Source: CAD feature listing. Evaluate the final solid. Frame: model axes, mm. Give positions to 0.01 mm unless a question says otherwise; leave off trailing zeros. Order: outer loops, then holes, each group sorted by start corner. A loop starts at its lowest first (then second) coordinate and runs counter-clockwise, first axis right, second up.
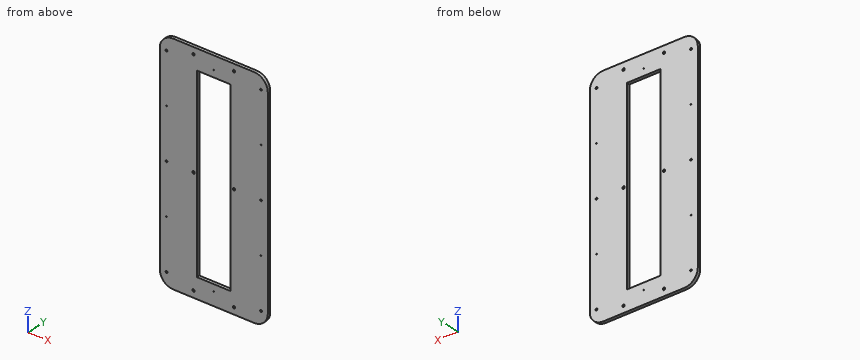
```python
from build123d import *

# Parameters (mm, degrees)
SKETCH1_W                = 203.2
SKETCH1_H                = 431.8
BOSS_EXTRUDE1_DEPTH      = 5.8
M4_CLEARANCE_HOLE1_D     = 4.5
M4_CLEARANCE_HOLE1_DEPTH = 12.7
M4_CLEARANCE_HOLE1_TIP   = 1.351936393
SKETCH7_W                = 63.5
SKETCH7_H                = 355.6
CUT_EXTRUDE2_DEPTH       = 478.257917692
FILLET1_R                = 25.4
M3_CLEARANCE_HOLE1_D     = 3.4
M3_CLEARANCE_HOLE1_DEPTH = 12.7
M3_CLEARANCE_HOLE1_TIP   = 1.021463052
SKETCH10_R               = 0.79375
CUT_EXTRUDE3_DEPTH       = 478.257917692


with BuildPart() as part:
    # Sketch1 → Boss-Extrude1 (new body)
    with BuildSketch(Plane(origin=(0, 0, 0), x_dir=(1, 0, 0), z_dir=(0, 1, 0))):
        with Locations((101.6, 215.9)):
            Rectangle(SKETCH1_W, SKETCH1_H)
    extrude(amount=BOSS_EXTRUDE1_DEPTH)

    # M4 Clearance Hole1
    with Locations(Plane(origin=(0, 5.8, 0), x_dir=(-1, 0, 0), z_dir=(0, 1, 0))):
        with Locations((-63.5, -419.1), (-139.7, -419.1), (-63.5, -215.9), (-139.7, -215.9), (-63.5, -12.7), (-139.7, -12.7)):
            Hole(M4_CLEARANCE_HOLE1_D / 2, depth=M4_CLEARANCE_HOLE1_DEPTH)
            with Locations((0, 0, -(M4_CLEARANCE_HOLE1_DEPTH + M4_CLEARANCE_HOLE1_TIP / 2))):  # 118° drill point
                Cone(0, M4_CLEARANCE_HOLE1_D / 2, M4_CLEARANCE_HOLE1_TIP, mode=Mode.SUBTRACT)

    # Sketch7 → Cut-Extrude2 (cut, through all)
    with BuildSketch(Plane(origin=(0, 5.8, 0), x_dir=(1, 0, 0), z_dir=(0, 1, 0))):
        with Locations((101.6, 215.9)):
            Rectangle(SKETCH7_W, SKETCH7_H)
    extrude(amount=-CUT_EXTRUDE2_DEPTH, mode=Mode.SUBTRACT)

    # Fillet1
    fillet1_edges = [part.edges().sort_by_distance(p)[0] for p in [
        (0, 2.9, -431.8),
        (203.2, 2.9, -431.8),
        (203.2, 2.9, 0),
        (0, 2.9, 0),
    ]]
    fillet(fillet1_edges, radius=FILLET1_R)

    # M3 Clearance Hole1
    with Locations(Plane(origin=(0, 5.8, 0), x_dir=(-1, 0, 0), z_dir=(0, 1, 0))):
        with Locations((-190.5, -406.4), (-190.5, -25.4), (-12.7, -25.4), (-12.7, -406.4), (-190.5, -215.9), (-12.7, -215.9)):
            Hole(M3_CLEARANCE_HOLE1_D / 2, depth=M3_CLEARANCE_HOLE1_DEPTH)
            with Locations((0, 0, -(M3_CLEARANCE_HOLE1_DEPTH + M3_CLEARANCE_HOLE1_TIP / 2))):  # 118° drill point
                Cone(0, M3_CLEARANCE_HOLE1_D / 2, M3_CLEARANCE_HOLE1_TIP, mode=Mode.SUBTRACT)

    # Sketch10 → Cut-Extrude3 (cut, through all)
    with BuildSketch(Plane(origin=(0, 5.8, 0), x_dir=(-1, 0, 0), z_dir=(0, 1, 0))):
        with Locations(Location((-190.5, -120.65, 0), (0, 0, 90))):
            Circle(SKETCH10_R)
        with Locations(Location((-12.7, -120.65, 0), (0, 0, 90))):
            Circle(SKETCH10_R)
        with Locations(Location((-101.6, -25.4, 0), (0, 0, 90))):
            Circle(SKETCH10_R)
        with Locations(Location((-101.6, -406.4, 0), (0, 0, 270))):
            Circle(SKETCH10_R)
        with Locations(Location((-12.7, -311.15, 0), (0, 0, 270))):
            Circle(SKETCH10_R)
        with Locations(Location((-190.5, -311.15, 0), (0, 0, 270))):
            Circle(SKETCH10_R)
    extrude(amount=-CUT_EXTRUDE3_DEPTH, mode=Mode.SUBTRACT)


solid = part.part
```
1) Material intervals for L1, parallel to X at y = 3.45, z = -406.4; L2, parallel to Z at x = 101.6, y = 2.65; L3, parallel to Z at x = 63.5, y = 2.8, sorted ascending.
Report:
L1: x = 0 to 11, 14.4 to 100.81, 102.39 to 188.8, 192.2 to 203.2
L2: z = -431.8 to -407.19, -405.61 to -393.7, -38.1 to -26.19, -24.61 to 0
L3: z = -431.8 to -421.35, -416.85 to -218.15, -213.65 to -14.95, -10.45 to 0
2) Section query A-A, the plane x = 91. Return the cut outline in (y, z).
Report:
outline: (0, -431.8) - (5.8, -431.8) - (5.8, -393.7) - (0, -393.7) - close; (0, -38.1) - (5.8, -38.1) - (5.8, 0) - (0, 0) - close
3) Section query B-B, the plane y = 1.85. Count the separate pieces of the cut face and the enclosed holes in it, and give its area (3 significant figures).
Report:
separate pieces: 1
enclosed holes: 19
area: 64,400 mm2
4) Section query C-C, the plane z = -353.5. Return the cut outline in (x, y).
Report:
outline: (0, 0) - (69.85, 0) - (69.85, 5.8) - (0, 5.8) - close; (133.35, 0) - (203.2, 0) - (203.2, 5.8) - (133.35, 5.8) - close
